```python
from build123d import *

# Parameters (mm, degrees)
SKETCH1_R                       = 15
BOSS_EXTRUDE1_DEPTH             = 6
BOSS_EXTRUDE2_REACH             = 8
BOSS_EXTRUDE2_DIRECTION_2_REACH = 8
SKETCH3_R                       = 4.5
CUT_EXTRUDE1_DEPTH              = 7
CUT_EXTRUDE1_DEPTH_BACK         = 7
CHAMFER1_SIZE                   = 1
SKETCH4_R                       = 1.6
CUT_EXTRUDE2_DEPTH              = 7
CUT_EXTRUDE2_DEPTH_BACK         = 7


with BuildPart() as part:
    # Sketch1 → Boss-Extrude1 (new body, symmetric)
    with BuildSketch(Plane.XY):
        Circle(SKETCH1_R)
    extrude(amount=BOSS_EXTRUDE1_DEPTH, both=True)

    # Boss-Extrude2: up to this face of the body (flat: up to its plane)
    boss_extrude2_end = Plane(part.part.faces().sort_by_distance((0, 0, 6))[0])
    # Sketch2 → Boss-Extrude2 (add, up to the picked face)
    with BuildSketch(Plane.XY, mode=Mode.PRIVATE) as boss_extrude2_sk1:
        with BuildLine():
            Line((-6, 20), (-6, 13.747727085))
            Line((-6, 13.747727085), (6, 13.747727085))
            Line((6, 13.747727085), (6, 20))
            ThreePointArc((6, 20), (0, 26), (-6, 20))
        make_face()
    boss_extrude2_tool1 = split(extrude(boss_extrude2_sk1.sketch, amount=BOSS_EXTRUDE2_REACH, mode=Mode.PRIVATE), bisect_by=boss_extrude2_end, keep=Keep.BOTH, mode=Mode.PRIVATE)
    add(boss_extrude2_tool1.solids().sort_by_distance((0, 19.311838, 0))[0])
    # Sketch2 → Boss-Extrude2 (add, up to the picked face)
    with BuildSketch(Plane.XY, mode=Mode.PRIVATE) as boss_extrude2_sk2:
        with BuildLine():
            Line((20.320508076, -4.803847577), (14.9058809, -1.67771112))
            Line((14.9058809, -1.67771112), (8.9058809, -12.070015965))
            Line((8.9058809, -12.070015965), (14.320508076, -15.196152423))
            ThreePointArc((14.320508076, -15.196152423), (22.516660498, -13), (20.320508076, -4.803847577))
        make_face()
    boss_extrude2_tool2 = split(extrude(boss_extrude2_sk2.sketch, amount=BOSS_EXTRUDE2_REACH, mode=Mode.PRIVATE), bisect_by=boss_extrude2_end, keep=Keep.BOTH, mode=Mode.PRIVATE)
    add(boss_extrude2_tool2.solids().sort_by_distance((16.724543, -9.655919, 0))[0])
    # Sketch2 → Boss-Extrude2 (add, up to the picked face)
    with BuildSketch(Plane.XY, mode=Mode.PRIVATE) as boss_extrude2_sk3:
        with BuildLine():
            Line((-14.320508076, -15.196152423), (-8.9058809, -12.070015965))
            Line((-8.9058809, -12.070015965), (-14.9058809, -1.67771112))
            Line((-14.9058809, -1.67771112), (-20.320508076, -4.803847577))
            ThreePointArc((-20.320508076, -4.803847577), (-22.516660498, -13), (-14.320508076, -15.196152423))
        make_face()
    boss_extrude2_tool3 = split(extrude(boss_extrude2_sk3.sketch, amount=BOSS_EXTRUDE2_REACH, mode=Mode.PRIVATE), bisect_by=boss_extrude2_end, keep=Keep.BOTH, mode=Mode.PRIVATE)
    add(boss_extrude2_tool3.solids().sort_by_distance((-16.724543, -9.655919, 0))[0])

    # Boss-Extrude2 direction 2: up to this face of the body (flat: up to its plane)
    boss_extrude2_direction_2_end = Plane(part.part.faces().sort_by_distance((0, 0, -6))[0])
    # Sketch2 → Boss-Extrude2 direction 2 (add, up to the picked face)
    with BuildSketch(Plane.XY, mode=Mode.PRIVATE) as boss_extrude2_direction_2_sk1:
        with BuildLine():
            Line((-6, 20), (-6, 13.747727085))
            Line((-6, 13.747727085), (6, 13.747727085))
            Line((6, 13.747727085), (6, 20))
            ThreePointArc((6, 20), (0, 26), (-6, 20))
        make_face()
    boss_extrude2_direction_2_tool1 = split(extrude(boss_extrude2_direction_2_sk1.sketch, amount=-BOSS_EXTRUDE2_DIRECTION_2_REACH, mode=Mode.PRIVATE), bisect_by=boss_extrude2_direction_2_end, keep=Keep.BOTH, mode=Mode.PRIVATE)
    add(boss_extrude2_direction_2_tool1.solids().sort_by_distance((0, 19.311838, 0))[0])
    # Sketch2 → Boss-Extrude2 direction 2 (add, up to the picked face)
    with BuildSketch(Plane.XY, mode=Mode.PRIVATE) as boss_extrude2_direction_2_sk2:
        with BuildLine():
            Line((20.320508076, -4.803847577), (14.9058809, -1.67771112))
            Line((14.9058809, -1.67771112), (8.9058809, -12.070015965))
            Line((8.9058809, -12.070015965), (14.320508076, -15.196152423))
            ThreePointArc((14.320508076, -15.196152423), (22.516660498, -13), (20.320508076, -4.803847577))
        make_face()
    boss_extrude2_direction_2_tool2 = split(extrude(boss_extrude2_direction_2_sk2.sketch, amount=-BOSS_EXTRUDE2_DIRECTION_2_REACH, mode=Mode.PRIVATE), bisect_by=boss_extrude2_direction_2_end, keep=Keep.BOTH, mode=Mode.PRIVATE)
    add(boss_extrude2_direction_2_tool2.solids().sort_by_distance((16.724543, -9.655919, 0))[0])
    # Sketch2 → Boss-Extrude2 direction 2 (add, up to the picked face)
    with BuildSketch(Plane.XY, mode=Mode.PRIVATE) as boss_extrude2_direction_2_sk3:
        with BuildLine():
            Line((-14.320508076, -15.196152423), (-8.9058809, -12.070015965))
            Line((-8.9058809, -12.070015965), (-14.9058809, -1.67771112))
            Line((-14.9058809, -1.67771112), (-20.320508076, -4.803847577))
            ThreePointArc((-20.320508076, -4.803847577), (-22.516660498, -13), (-14.320508076, -15.196152423))
        make_face()
    boss_extrude2_direction_2_tool3 = split(extrude(boss_extrude2_direction_2_sk3.sketch, amount=-BOSS_EXTRUDE2_DIRECTION_2_REACH, mode=Mode.PRIVATE), bisect_by=boss_extrude2_direction_2_end, keep=Keep.BOTH, mode=Mode.PRIVATE)
    add(boss_extrude2_direction_2_tool3.solids().sort_by_distance((-16.724543, -9.655919, 0))[0])

    # Sketch3 → Cut-Extrude1 (cut, two sides)
    with BuildSketch(Plane.XY) as cut_extrude1_sk:
        Circle(SKETCH3_R)
    extrude(amount=CUT_EXTRUDE1_DEPTH, mode=Mode.SUBTRACT)
    extrude(cut_extrude1_sk.sketch, amount=-CUT_EXTRUDE1_DEPTH_BACK, mode=Mode.SUBTRACT)

    # Chamfer1
    chamfer1_edges = [part.edges().sort_by_distance(p)[0] for p in [
        (12.990381057, 7.5, -6),
        (12.990381057, 7.5, 6),
        (11.613194488, -13.633084194, 6),
        (22.516660498, -13, 6),
        (17.613194488, -3.240779349, 6),
        (11.613194488, -13.633084194, -6),
        (17.613194488, -3.240779349, -6),
        (22.516660498, -13, -6),
        (0, -15, -6),
        (0, -15, 6),
        (-17.613194488, -3.240779349, 6),
        (-22.516660498, -13, 6),
        (-11.613194488, -13.633084194, 6),
        (-17.613194488, -3.240779349, -6),
        (-11.613194488, -13.633084194, -6),
        (-22.516660498, -13, -6),
        (-4.5, 0, -6),
        (-4.5, 0, 6),
        (-12.990381057, 7.5, -6),
        (-12.990381057, 7.5, 6),
        (6, 16.873863542, 6),
        (0, 26, 6),
        (-6, 16.873863542, 6),
        (6, 16.873863542, -6),
        (-6, 16.873863542, -6),
        (0, 26, -6),
    ]]
    chamfer(chamfer1_edges, length=CHAMFER1_SIZE)

    # Sketch4 → Cut-Extrude2 (cut, two sides)
    with BuildSketch(Plane.XY) as cut_extrude2_sk:
        with Locations((0, 20)):
            Circle(SKETCH4_R)
        with Locations((17.320508076, -10)):
            Circle(SKETCH4_R)
        with Locations((-17.320508076, -10)):
            Circle(SKETCH4_R)
    extrude(amount=CUT_EXTRUDE2_DEPTH, mode=Mode.SUBTRACT)
    extrude(cut_extrude2_sk.sketch, amount=-CUT_EXTRUDE2_DEPTH_BACK, mode=Mode.SUBTRACT)


solid = part.part
```
Build history of the part. All positions in model axes, mm. A direction names the side the tool comes from. Round coordinates to 2 decimals unless told otherwise and drop trailing zeros. Loops run counter-clockwise (first coordinate to the right, second up) from the corner with the lowest first, then second, coordinate; pieces in that order, holes last.
Item 1: Drill centre lines: line 1 along Y through (x, z) = (0, 2.5); line 2 along X through (y, z) = (20, 1); line 3 along Y through (x, z) = (3.5, -1.25). Where is each one in solid material? Low to high.
Item 2: Pin check, flat tips, straight feed: P1, Ø1.5, axis at y = 0.5, z = 2, coming from the -X side; P2, Ø5, axis at x = -13.5, z = 3.5, coming from the +Y side; P3, Ø2, axis at y = 12, z = 2, coming from the +X side; P4, Ø1.9, axis at x = -17.32, y = -10, coming from the -Z side. Stop position of each tip, or through.
Item 3: Two-plate mould, pull along X, no slides. Class faces 6 (the face through (-11.651, -13.655, 0.07)), 7 (the face through (5, -4, 6)), 8 (the face through (-5.5, 16.6, 5.5)), 9 (the face through (0, -15, 0)): released by +X, released by -X, zero draft, split by the parting line, or undercut.
Item 4: Saw through at B-B (y = -10). List the corners of the cut face in (x, z), then the cut area to 3 significant figures.
Item 5: Saw through at C-C (z = -2). List the corners of the cut face in (x, y), then the cut area to 3 significant figures.
Item 6: Saw through at A-A (x = 0). List the corners of the cut face in (y, z).
Item 7: Which spindle directions (+Z, -Z, +X, -X, +Y, -Y) get a long thin tool onto all of the face, cutting with end or side? Do faces 1 (the face through (6, 17, 0)), 2 (the face through (-11.611, -13.063, 5.493)), 3 (the face through (11.575, -13.611, 0.07)), 4 (the face through (5.5, 16.5, 5.5)), 5 (the face through (-5.5, 16.6, -5.5)). Say none if no direction does.
Worked answers:
1. line 1: y = -15 to -4.5, 4.5 to 18.4, 21.6 to 26
1. line 2: x = -6 to -1.6, 1.6 to 6
1. line 3: y = -14.59 to -2.83, 2.83 to 24.87
2. P1: stops at x = -15
2. P2: stops at y = 10.2
2. P3: stops at x = 10.2
2. P4: passes through
3. face 6: undercut
3. face 7: zero draft
3. face 8: released by -X
3. face 9: undercut
4. outline: (-23.32, -5) - (-22.32, -6) - (-18.92, -6) - (-18.92, 6) - (-22.32, 6) - (-23.32, 5) - close; (-15.72, -6) - (15.72, -6) - (15.72, 6) - (-15.72, 6) - close; (18.92, -6) - (22.32, -6) - (23.32, -5) - (23.32, 5) - (22.32, 6) - (18.92, 6) - close
4. area: 481 mm2
5. outline: (-20.32, -4.8) arc R6 ccw to (-14.32, -15.2) - (-8.91, -12.07) arc R15 ccw to (8.91, -12.07) - (14.32, -15.2) arc R6 ccw to (20.32, -4.8) - (14.91, -1.68) arc R15 ccw to (6, 13.75) - (6, 20) arc R6 ccw to (-6, 20) - (-6, 13.75) arc R15 ccw to (-14.91, -1.68) - close; hole circle Ø3.2 at (-17.32, -10); hole circle Ø9 at (0, 0); hole circle Ø3.2 at (0, 20); hole circle Ø3.2 at (17.32, -10)
5. area: 984 mm2
6. outline: (-15, -5) - (-14, -6) - (-5.5, -6) - (-4.5, -5) - (-4.5, 5) - (-5.5, 6) - (-14, 6) - (-15, 5) - close; (4.5, -5) - (5.5, -6) - (18.4, -6) - (18.4, 6) - (5.5, 6) - (4.5, 5) - close; (21.6, -6) - (25, -6) - (26, -5) - (26, 5) - (25, 6) - (21.6, 6) - close
7. face 1: +Z, -Z, +X, +Y
7. face 2: +Z, -Y
7. face 3: +Z, -Z, -Y
7. face 4: +Z, +X, +Y
7. face 5: -Z, -X, +Y
